Could you check a few things on this drawing? It's one solid part, dimensions in mm from its lowest x, y, z. A direction names the side the tool comes from. Round coordinates to 2 decimals unless told otherwise and drop trailing zeros. Order: outer loops, then holes, each group sorted by start corner. A loop starts at its lowest first (then second) coordinate and runs counter-clockwise, first axis right, second up. Notation, with made-up numbers: (68, -23) -> (85, -23) arc R20 cw to (85, -1) -> close; hole circle Ø5 at (31.25, 44). An arc over 180 degrees is marked (long way). Use a Markdown table: item, result. Add a question column.
(1) I want a section at C-C, the plane z = 2. Please give me the cut outline in (x, y) (1 decimal), then the cut area to 3 significant figures.
(2) I want a section at A-A, the plane z = 6.25. Please give me the cut outline in (x, y) (1 decimal).
(3) I want a section at B-B, the plane y = 1.6. Please give me the cut outline in (x, z) (1 decimal).
(4) If I drill on probe 1 along Z at (x, y) = (24, 1.7); probe 2 along Z at (x, y) = (26, 0.25) (1 decimal); probe 3 along X at (y, z) = (2.9, 5.25) (1 decimal), over which ranges is the centre line in solid material (lowest first)?
(5) On a 3-axis mill with a long thin cutter (end or side, diameter ignored), from which of +Z, -Z, +X, -X, +Y, -Y can I reach the whole of each face in a straight line? I mean the marked faces 1 and 2. Say none if no direction works.
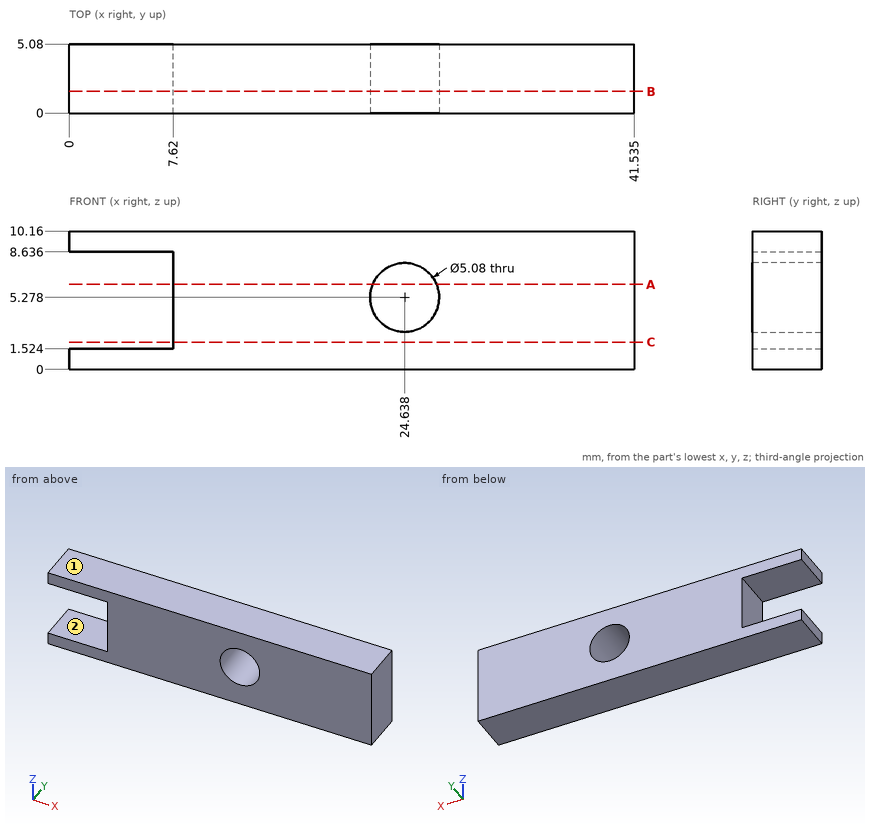
Taken from the geometry:
| question | item | result |
|---|---|---|
| 1 | outline | (7.6, 0) -> (41.5, 0) -> (41.5, 5.1) -> (7.6, 5.1) -> close |
| 1 | area | 172 mm2 |
| 2 | outline | (7.6, 0) -> (22.3, 0) -> (22.3, 5.1) -> (7.6, 5.1) -> close; (27, 0) -> (41.5, 0) -> (41.5, 5.1) -> (27, 5.1) -> close |
| 3 | outline | (0, 0) -> (41.5, 0) -> (41.5, 10.2) -> (0, 10.2) -> (0, 8.6) -> (7.6, 8.6) -> (7.6, 1.5) -> (0, 1.5) -> close; hole circle Ø5.1 at (24.6, 5.3) |
| 4 | probe 1 | z = 0 to 2.82, 7.74 to 10.16 |
| 4 | probe 2 | z = 0 to 3.1, 7.4 to 10.2 |
| 4 | probe 3 | x = 7.6 to 22.1, 27.2 to 41.5 |
| 5 | face 1 | +Z, +X, -X, +Y, -Y |
| 5 | face 2 | -X, +Y, -Y |
